Autodesk Inventor part; units mm, degrees
ref_plane "YZ Plane" through (0, 0, 0) normal (1, 0, 0) x (0, 1, 0)
ref_plane "XZ Plane" through (0, 0, 0) normal (0, 1, 0) x (-1, 0, 0)
ref_plane "XY Plane" through (0, 0, 0) normal (0, 0, 1) x (1, 0, 0)
sketch "Szkic1" plane through (0, 0, 0) normal (0, 1, 0) x (-1, 0, 0)
  line L0 (5.43, 11.8473) -> (13.43, 11.8473)
  line L1 (13.43, -12.1527) -> (-9.57, -12.1527)
  line L2 (-9.57, -12.1527) -> (-9.57, -27.1527)
  line L3 (-9.57, -27.1527) -> (-21.17, -27.1527)
  arc A0 (5.43, 11.8473) -> (3.5548, 10.5426) centre (5.43, 9.8473) ccw
  line L4 (3.5548, 10.5426) -> (-8.7625, -5.2144)
  arc A1 (-12.3382, -3.9827) -> (-8.7625, -5.2144) centre (-10.3382, -3.9827) ccw
  line L5 (-12.3382, -3.9827) -> (-12.3382, 0.0173)
  line L6 (-21.17, -27.1527) -> (-21.17, 0.0173)
  line L7 (-21.17, 0.0173) -> (-12.3382, 0.0173)
  line L8 (13.43, 11.8473) -> (13.43, 5.8473)
  line L9 (13.43, 5.8473) -> (9.43, 5.8473)
  line L10 (9.43, 5.8473) -> (9.43, 1.8473)
  line L11 (9.43, 1.8473) -> (13.43, 1.8473)
  line L12 (13.43, 1.8473) -> (13.43, -1.1527)
  line L13 (13.43, 1.8473) -> (13.43, -2.1527)
  line L14 (13.43, -2.1527) -> (9.43, -2.1527)
  line L15 (9.43, -2.1527) -> (9.43, -6.1527)
  line L16 (9.43, -6.1527) -> (13.43, -6.1527)
  line L17 (13.43, -6.1527) -> (13.43, -12.1527)
  point P0 (0, 0)
  dimension "d0" = 8
  dimension "d1" = 24
  dimension "d2" = 23
  dimension "d3" = 15
  dimension "d4" = 11.6
  dimension "d5" = 2
  dimension "d6" = 20
  dimension "d7" = 2
  dimension "d8" = 4
  dimension "d16" = 6
  dimension "d17" = 4
  dimension "d18" = 4
  dimension "d19" = 4
  dimension "d21" = 4
  dimension "d22" = 4
  dimension "d23" = 4
  dimension "d24" = 4
revolve "Obrót1" add sketch "Szkic1" angle 360 about axis through (21.17, 0, -27.1527) along (0, 0, 1)
sketch "Szkic2" plane through (21.17, 0, -27.1527) normal (0, 0, -1) x (-1, 0, 0)
  point P0 (21.17, 0)
sketch "Szkic3" plane through (21.17, 0, -27.1527) normal (0, 0, -1) x (-1, 0, 0)
  circle A0 centre (0, 0) radius 6
  point P0 (21.17, 0)
  dimension "d13" = 12
extrude "Wyciągnięcie proste2" cut sketch "Szkic3" against normal blind 39
properties part number "7Tłok" material "Tworzywo sztuczne PET"
Input: part model. Units: mm. Frame: model coordinates. A direction names the side the tool comes from. Coordinates: 2 decimals unless noted, no trailing zeros. Loops run counter-clockwise (first coordinate to the right, second up) from the corner with the lowest first, then second, coordinate; pieces in that order, holes last. Notation, with made-up numbers: M -34.75,-9.75 L -3.75,-9.75 A25 cw -3.75,29.25 Z; hole C 52,6.25 d5. An arc over 180 degrees is marked long. Use a Markdown table: item, result. Add a question column.
1) Section C-C, the plane x = -6.5. Return the cut outline in (y, z).
2) Section D-D, the plane z = -24. Return the cut outline in (x, y), plus the area to 3 significant figures.
3) Draft query along Z for faces 4 (the flat face through (19, 31, -2.153)), 5 (the flat face through (11, 25, 11.847)), 6 (the flat face through (19, 31, -6.153)), 7 (the cylindrical face through (10.106, 3.484, -19.758)). Return one class per face: +Z half, -Z half, draft (parallel to the pull), parting line (faces both ways), or undercut.
4) Section B-B, the plane z = -11. Return the cut outline in (x, y), plus the area to 3 significant figures.
5) Section A-A, the plane y = -28.5. Return the cut outline in (x, z).
6) Set-up query: faces 1 (the flat face through (15, 2, 0.017)), 2 (the flat face through (19, 31, 5.847)), 3 (the flat face through (6, 0, -12.153)). Return all of +Z, -Z, +X, -X, +Y, -Y with unobstructed straight access to the full face (end or side cutting, diameter ignored); none if empty.
7) Pin query (flat end, axial travel): P1, Ø4, axis at x = 34.5, z = 0.5, coming from the -Y side; P2, Ø10, axis at y = 16, z = -1, coming from the -X side; P3, Ø14, axis at x = 18, y = 2, coming from the +Z side. Return the tip coordinate at first contact, or that it passes through.
8) Line query: L1, parallel to Z at x = 52, y = 13.5; L2, parallel to Y at x = 21, z = -14; L3, parallel to Y at x = 21.17, z = -7.75. Output: solid intervals per line, ascending. Write a range as from..to.
Answer below:
| question | item | result |
|---|---|---|
| 1 | outline | M -20.77,-12.15 L 20.77,-12.15 L 20.77,-6.15 L 13.07,-6.15 L 13.07,-2.15 L 20.77,-2.15 L 20.77,1.85 L 13.07,1.85 L 13.07,5.85 L 20.77,5.85 L 20.77,11.85 L -20.77,11.85 L -20.77,5.85 L -13.07,5.85 L -13.07,1.85 L -20.77,1.85 L -20.77,-2.15 L -13.07,-2.15 L -13.07,-6.15 L -20.77,-6.15 Z |
| 2 | outline | C 21.17,0 d23.2; hole C 21.17,0 d12 |
| 2 | area | 310 mm2 |
| 3 | face 4 | undercut |
| 3 | face 5 | +Z half |
| 3 | face 6 | undercut |
| 3 | face 7 | draft |
| 4 | outline | C 21.17,0 d69.2; hole C 21.17,0 d12 |
| 4 | area | 3,650 mm2 |
| 5 | outline | M 1.55,-12.15 L 40.79,-12.15 L 40.79,-6.15 L 32.31,-6.15 L 32.31,-2.15 L 40.79,-2.15 L 40.79,1.85 L 32.31,1.85 L 32.31,5.85 L 40.79,5.85 L 40.79,11.85 L 1.55,11.85 L 1.55,5.85 L 10.03,5.85 L 10.03,1.85 L 1.55,1.85 L 1.55,-2.15 L 10.03,-2.15 L 10.03,-6.15 L 1.55,-6.15 Z |
| 6 | face 1 | +Z |
| 6 | face 2 | none |
| 6 | face 3 | -Z |
| 7 | P1 | y = -32.69 |
| 7 | P2 | x = -11.63 |
| 7 | P3 | z = 0.02 |
| 8 | L1 | -12.15..-6.15, -2.15..1.85, 5.85..11.85 |
| 8 | L2 | -11.6..-6, 6..11.6 |
| 8 | L3 | -34.6..-6, 6..34.6 |
